The listing builds one solid part. Answer for the finished solid, in the listing's coordinates (mm). A direction names the side the tool comes from. Round coordinates to 2 decimals unless told otherwise and drop trailing zeros. Loops run counter-clockwise (first coordinate to the right, second up) from the corner with the lowest first, then second, coordinate; pieces in that order, holes last. Notation, with made-up numbers: (79.25, -12) - (135.25, -12) arc R11 cw to (135.25, -8) - close; hole circle Ø9 at (67.5, -39.75). An arc over 180 degrees is marked (long way). Write item = value, one per line. Start each with the question number.
1) Section A-A, the plane z = 15 is taken. Give the number of separate pieces and of enclosed holes in the cut face, and give its area (3 significant figures).
2) A tool of negligible diameter and unlimited length cuts with its end or side. For faces 1 (the cylindrical face through (-19, -24, 25)), 2 (the flat face through (-2, 82.5, 22)), from which of +Z, -Z, +X, -X, +Y, -Y can it reach the whole face along a straight path? Write none if from no direction.
3) For a pull along X with two mould halves and no side action, classify faces 3 (the flat face through (19, -32, 40)), 4 (the cylindrical face through (142.51, -72.24, 24.72)), 5 (the flat face through (1, 78, 5)) as released by +X, released by -X, zero draft, split by the parting line, or undercut.
4) Given pin 1 Ø2 at (x, y) = (30, -9.5) entering from -Z; pin 2 Ø2.5 at (y, z) = (-79, 37) entering from +X; pin 3 Ø2 at (x, y) = (-18, -31.5) entering from -Z; pin 4 Ø4 at (x, y) = (-149, -41.5) entering from +Z, each flat-ended and moving along its own axis, determine where each tip first touches the part or whether it passes through.
5) Section B-B, the plane x = -4.5 is taken. Determine the outline of the cut face in (y, z), and give its area (3 significant figures).
6) Straight lines are drawn through the part: line 1 along Y through (x, z) = (130, 20.5); line 2 along Y through (x, z) = (-51.5, 15.5); line 3 along X through (y, z) = (-10, 43). For each, find the intervals that lie inside material, in ascending order.
7) Section C-C, the plane y = -3.5 is taken. Determine the outline of the cut face in (x, z), and give its area (3 significant figures).
from build123d import *

# Parameters (mm, degrees)
EXTRUDE_1_DEPTH      = 50
SKETCH_1_4_R         = 5.1
CUT_EXTRUDE_1_DEPTH  = 45
CUT_EXTRUDE_2_DEPTH  = 5
SKETCH_1_6_R         = 5.1
CUT_EXTRUDE_3_DEPTH  = 5
SKETCH_1_7_R         = 2.6
CUT_EXTRUDE_4_DEPTH  = 25
FILLET_2_R           = 5
SKETCH_14_R          = 1.6
SKETCH_14_W          = 14
SKETCH_14_H          = 9
USB_DEPTH            = 5
SKETCH_16_W          = 24
SKETCH_16_H          = 24
CUT_EXTRUDE_12_DEPTH = 5
SKETCH_18_W          = 24
SKETCH_18_H          = 24
CUT_EXTRUDE_13_DEPTH = 5
EXTRUDE_2_DEPTH      = 40
EXTRUDE_3_DEPTH      = 2
SKETCH_29_4_R        = 2.95
SKETCH_29_4_R_2      = 1.25
EXTRUDE_4_DEPTH      = 5
SKETCH_29_5_R        = 3.3
SKETCH_29_5_R_2      = 1.3
EXTRUDE_5_DEPTH      = 6.5


with BuildPart() as part:
    # Sketch 1 → Extrude 1 (new body)
    with BuildSketch(Plane.XY):
        with BuildLine():
            Line((-130, 82.5), (130, 82.5))
            ThreePointArc((130, 82.5), (145.909902577, 75.909902577), (152.5, 60))
            Line((152.5, 60), (152.5, -60))
            ThreePointArc((152.5, -60), (145.909902577, -75.909902577), (130, -82.5))
            Line((130, -82.5), (-130, -82.5))
            ThreePointArc((-130, -82.5), (-145.909902577, -75.909902577), (-152.5, -60))
            Line((-152.5, -60), (-152.5, 60))
            ThreePointArc((-152.5, 60), (-145.909902577, 75.909902577), (-130, 82.5))
        make_face()
    extrude(amount=EXTRUDE_1_DEPTH)

    # Sketch 1_4 → Cut-Extrude 1 (cut)
    with BuildSketch(Plane.XY):
        with BuildLine():
            Line((-130, 77.5), (130, 77.5))
            ThreePointArc((130, 77.5), (142.374368671, 72.374368671), (147.5, 60))
            Line((147.5, 60), (147.5, -60))
            ThreePointArc((147.5, -60), (142.374368671, -72.374368671), (130, -77.5))
            Line((130, -77.5), (-130, -77.5))
            ThreePointArc((-130, -77.5), (-142.374368671, -72.374368671), (-147.5, -60))
            Line((-147.5, -60), (-147.5, 60))
            ThreePointArc((-147.5, 60), (-142.374368671, 72.374368671), (-130, 77.5))
        make_face()
        with Locations(Location((130, 60, 0), (0, 0, 180))):
            Circle(SKETCH_1_4_R, mode=Mode.SUBTRACT)
        with Locations(Location((130, -60, 0), (0, 0, 180))):
            Circle(SKETCH_1_4_R, mode=Mode.SUBTRACT)
        with Locations(Location((-130, 60, 0), (0, 0, 180))):
            Circle(SKETCH_1_4_R, mode=Mode.SUBTRACT)
        with Locations(Location((-130, -60, 0), (0, 0, 180))):
            Circle(SKETCH_1_4_R, mode=Mode.SUBTRACT)
    extrude(amount=CUT_EXTRUDE_1_DEPTH, mode=Mode.SUBTRACT)

    # Sketch 1_5 → Cut-Extrude 2 (cut)
    with BuildSketch(Plane.XY):
        with BuildLine():
            ThreePointArc((-150.2, 60), (-144.28355698, 74.28355698), (-130, 80.2))
            Line((-130, 80.2), (130, 80.2))
            ThreePointArc((130, 80.2), (144.28355698, 74.28355698), (150.2, 60))
            Line((150.2, 60), (150.2, -60))
            ThreePointArc((150.2, -60), (144.28355698, -74.28355698), (130, -80.2))
            Line((130, -80.2), (-130, -80.2))
            ThreePointArc((-130, -80.2), (-144.28355698, -74.28355698), (-150.2, -60))
            Line((-150.2, -60), (-150.2, 60))
        make_face()
        with BuildLine():
            Line((-147.5, 60), (-147.5, -60))
            ThreePointArc((-147.5, -60), (-142.374368671, -72.374368671), (-130, -77.5))
            Line((-130, -77.5), (130, -77.5))
            ThreePointArc((130, -77.5), (142.374368671, -72.374368671), (147.5, -60))
            Line((147.5, -60), (147.5, 60))
            ThreePointArc((147.5, 60), (142.374368671, 72.374368671), (130, 77.5))
            Line((130, 77.5), (-130, 77.5))
            ThreePointArc((-130, 77.5), (-142.374368671, 72.374368671), (-147.5, 60))
        make_face(mode=Mode.SUBTRACT)
    extrude(amount=CUT_EXTRUDE_2_DEPTH, mode=Mode.SUBTRACT)

    # Sketch 1_6 → Cut-Extrude 3 (cut)
    with BuildSketch(Plane.XY):
        with Locations(Location((130, 60, 0), (0, 0, 180))):
            Circle(SKETCH_1_6_R)
        with Locations(Location((130, -60, 0), (0, 0, 180))):
            Circle(SKETCH_1_6_R)
        with Locations(Location((-130, 60, 0), (0, 0, 180))):
            Circle(SKETCH_1_6_R)
        with Locations(Location((-130, -60, 0), (0, 0, 180))):
            Circle(SKETCH_1_6_R)
    extrude(amount=CUT_EXTRUDE_3_DEPTH, mode=Mode.SUBTRACT)

    # Sketch 1_7 → Cut-Extrude 4 (cut)
    with BuildSketch(Plane.XY):
        with Locations((-130, -60)):
            Circle(SKETCH_1_7_R)
        with Locations((130, 60)):
            Circle(SKETCH_1_7_R)
        with Locations((130, -60)):
            Circle(SKETCH_1_7_R)
        with Locations((-130, 60)):
            Circle(SKETCH_1_7_R)
    extrude(amount=CUT_EXTRUDE_4_DEPTH, mode=Mode.SUBTRACT)

    # Fillet 2
    fillet_2_edges = [part.edges().sort_by_distance(p)[0] for p in [
        (152.5, 0, 50),
        (145.909902577, 75.909902577, 50),
        (0, 82.5, 50),
        (-145.909902577, 75.909902577, 50),
        (-152.5, 0, 50),
        (-145.909902577, -75.909902577, 50),
        (0, -82.5, 50),
        (145.909902577, -75.909902577, 50),
    ]]
    fillet(fillet_2_edges, radius=FILLET_2_R)

    # Sketch 14 → USB (cut)
    with BuildSketch(Plane.XZ.offset(82.5)):
        with Locations(Location((-71, 38, 0), (0, 0, 270))):
            Circle(SKETCH_14_R)
        with Locations(Location((-89, 38, 0), (0, 0, 270))):
            Circle(SKETCH_14_R)
        with Locations((-80, 38)):
            Rectangle(SKETCH_14_W, SKETCH_14_H)
    extrude(amount=-USB_DEPTH, mode=Mode.SUBTRACT)

    # Sketch 16 → Cut-Extrude 12 (cut)
    with BuildSketch(Plane(origin=(152.5, 0, 0), x_dir=(0, 0, -1), z_dir=(1, 0, 0))):
        with Locations((-30, -38)):
            Rectangle(SKETCH_16_W, SKETCH_16_H)
    extrude(amount=-CUT_EXTRUDE_12_DEPTH, mode=Mode.SUBTRACT)

    # Sketch 18 → Cut-Extrude 13 (cut)
    with BuildSketch(Plane.ZY.offset(152.5)):
        with Locations((30, -38)):
            Rectangle(SKETCH_18_W, SKETCH_18_H)
    extrude(amount=-CUT_EXTRUDE_13_DEPTH, mode=Mode.SUBTRACT)

    # Sketch 19 → Extrude 2 (add)
    with BuildSketch(Plane(origin=(0, 0, 45), x_dir=(-1, 0, 0), z_dir=(0, 0, -1))):
        with BuildLine():
            Line((-103, 40), (-18, 40))
            ThreePointArc((-18, 40), (-14, 36), (-18, 32))
            Line((-18, 32), (-103, 32))
            ThreePointArc((-103, 32), (-107, 36), (-103, 40))
        make_face()
        with BuildLine():
            Line((103, 40), (18, 40))
            ThreePointArc((18, 40), (14, 36), (18, 32))
            Line((18, 32), (103, 32))
            ThreePointArc((103, 32), (107, 36), (103, 40))
        make_face()
        with BuildLine():
            Line((-103, -20), (-23, -20))
            ThreePointArc((-23, -20), (-19, -24), (-23, -28))
            Line((-23, -28), (-103, -28))
            ThreePointArc((-103, -28), (-107, -24), (-103, -20))
        make_face()
        with BuildLine():
            Line((103, -20), (23, -20))
            ThreePointArc((23, -20), (19, -24), (23, -28))
            Line((23, -28), (103, -28))
            ThreePointArc((103, -28), (107, -24), (103, -20))
        make_face()
    extrude(amount=EXTRUDE_2_DEPTH)

    # Sketch 29 → Extrude 3 (add)
    with BuildSketch(Plane(origin=(0, 0, 45), x_dir=(-1, 0, 0), z_dir=(0, 0, -1))):
        Polygon((-14.35, -45.2), (14.35, -45.2), (14.35, -18.5), (12.85, -18.5), (12.85, -20), (12.85, -43.7), (-12.85, -43.7), (-12.85, -20), (-12.85, -18.5), (-14.35, -18.5), align=None)
    extrude(amount=EXTRUDE_3_DEPTH)

    # Sketch 29_4 → Extrude 4 (add)
    # profile 1 of 2: a face of its own
    with BuildSketch(Plane(origin=(0, 0, 45), x_dir=(-1, 0, 0), z_dir=(0, 0, -1))):
        with Locations(Location((-17.5, -31.85, 0), (0, 0, 180))):
            Circle(SKETCH_29_4_R)
        with Locations((-17.5, -31.85)):
            Circle(SKETCH_29_4_R_2, mode=Mode.SUBTRACT)
    # profile 2 of 2: a face of its own
    with BuildSketch(Plane(origin=(0, 0, 45), x_dir=(-1, 0, 0), z_dir=(0, 0, -1))):
        with Locations((17.5, -31.85)):
            Circle(SKETCH_29_4_R)
        with Locations(Location((17.5, -31.85, 0), (0, 0, 180))):
            Circle(SKETCH_29_4_R_2, mode=Mode.SUBTRACT)
    extrude(amount=EXTRUDE_4_DEPTH)

    # Sketch 29_5 → Extrude 5 (add)
    # profile 1 of 4: a face of its own
    with BuildSketch(Plane(origin=(0, 0, 45), x_dir=(-1, 0, 0), z_dir=(0, 0, -1))):
        with Locations(Location((-30, 20, 0), (0, 0, 180))):
            Circle(SKETCH_29_5_R)
        with Locations(Location((-30, 20, 0), (0, 0, 180))):
            Circle(SKETCH_29_5_R_2, mode=Mode.SUBTRACT)
    # profile 2 of 4: a face of its own
    with BuildSketch(Plane(origin=(0, 0, 45), x_dir=(-1, 0, 0), z_dir=(0, 0, -1))):
        with Locations(Location((-30, -10, 0), (0, 0, 180))):
            Circle(SKETCH_29_5_R)
        with Locations(Location((-30, -10, 0), (0, 0, 180))):
            Circle(SKETCH_29_5_R_2, mode=Mode.SUBTRACT)
    # profile 3 of 4: a face of its own
    with BuildSketch(Plane(origin=(0, 0, 45), x_dir=(-1, 0, 0), z_dir=(0, 0, -1))):
        with Locations(Location((30, 20, 0), (0, 0, 180))):
            Circle(SKETCH_29_5_R)
        with Locations(Location((30, 20, 0), (0, 0, 180))):
            Circle(SKETCH_29_5_R_2, mode=Mode.SUBTRACT)
    # profile 4 of 4: a face of its own
    with BuildSketch(Plane(origin=(0, 0, 45), x_dir=(-1, 0, 0), z_dir=(0, 0, -1))):
        with Locations(Location((30, -10, 0), (0, 0, 180))):
            Circle(SKETCH_29_5_R)
        with Locations(Location((30, -10, 0), (0, 0, 180))):
            Circle(SKETCH_29_5_R_2, mode=Mode.SUBTRACT)
    extrude(amount=EXTRUDE_5_DEPTH)


solid = part.part
Geometry check:
q1.separate_pieces = 9
q1.enclosed_holes = 5
q1.area = 7,510 mm2
q2.face_1 = -Z
q2.face_2 = +Z, -Z, +X, -X, +Y
q3.face_3 = zero draft
q3.face_4 = undercut
q3.face_5 = undercut
q4.pin_1 = 38.5
q4.pin_2 = 143.83
q4.pin_3 = 40
q4.pin_4 = 50
q5.outline = (-82.5, 0) - (-80.2, 0) - (-80.2, 5) - (-77.5, 5) - (-77.5, 45) - (-45.2, 45) - (-45.2, 43) - (-43.7, 43) - (-43.7, 45) - (77.5, 45) - (77.5, 5) - (80.2, 5) - (80.2, 0) - (82.5, 0) - (82.5, 45) arc R5 ccw to (77.5, 50) - (-77.5, 50) arc R5 ccw to (-82.5, 45) - close
q5.area = 1,240 mm2
q6.line_1 = -82.5 to -77.5, -65.1 to -62.6, -57.4 to -54.9, 54.9 to 57.4, 62.6 to 65.1, 77.5 to 82.5
q6.line_2 = -82.5 to -77.5, -28 to -20, 32 to 40, 77.5 to 82.5
q6.line_3 = -152.5 to -147.5, -33.3 to -31.3, -28.7 to -26.7, 26.7 to 28.7, 31.3 to 33.3, 147.5 to 152.5
q7.outline = (-152.5, 0) - (-150.2, 0) - (-150.2, 5) - (-147.5, 5) - (-147.5, 45) - (147.5, 45) - (147.5, 5) - (150.2, 5) - (150.2, 0) - (152.5, 0) - (152.5, 45) arc R5 ccw to (147.5, 50) - (-147.5, 50) arc R5 ccw to (-152.5, 45) - close
q7.area = 1,940 mm2
